Autodesk Inventor part; units mm, degrees
ref_plane "YZ Plane" through (0, 0, 0) normal (1, 0, 0) x (0, 1, 0)
ref_plane "XZ Plane" through (0, 0, 0) normal (0, 1, 0) x (-1, 0, 0)
ref_plane "XY Plane" through (0, 0, 0) normal (0, 0, 1) x (1, 0, 0)
sketch "Sketch1" plane through (0, 0, 0) normal (0, 1, 0) x (-1, 0, 0)
  line L0 (40, 40) -> (-40, 40) construction
  line L1 (-40, 40) -> (-40, -40) construction
  line L2 (-40, -40) -> (40, -40) construction
  line L3 (40, -40) -> (40, 40) construction
  line L4 (-40, 40) -> (40, -40) construction
  line L5 (100, -45) -> (-100, -45)
  line L6 (-100, -45) -> (-100, 100)
  line L7 (-100, 100) -> (100, 100)
  line L8 (100, 100) -> (100, -45)
  circle A0 centre (85, 0) radius 6.5
  circle A1 centre (0, 85) radius 6.5
  circle A2 centre (-85, 0) radius 6.5
  line L9 (0, 40) -> (0, -40) construction
  line L10 (100, 15) -> (20, 100)
  line L11 (-20, 100) -> (-100, 15)
  line L12 (100, -15) -> (71.7647, -45)
  line L13 (-100, -15) -> (-71.7647, -45)
  line L14 (0, 0) -> (-40, 0) construction
  point P0 (0, 0)
  point P1 (0, 0)
  dimension "d2" = 80
  dimension "d3" = 80
  dimension "d17" = 5
  dimension "d18" = 13
  dimension "d19" = 45
  dimension "d20" = 45
  dimension "d21" = 40
  dimension "d22" = 15
  dimension "d23" = 15
  dimension "d24" = 30
extrude "Plate1" add sketch "Sketch1" along normal blind 3 contours L5 L13 L6 L11 L7 L10 L8 L12
fillet "Corner Round2" radius 6 8 edges at (-20, 1.5, 100) (20, 1.5, 100) (100, 1.5, 15) (100, 1.5, -15) (71.7647, 1.5, -45) (-100, 1.5, 15) (-100, 1.5, -15) (-71.7647, 1.5, -45)
equation "\"d20\" = d19"
equation "\"d23\" = d22"
equation "\"BendReliefWidth\" = Thickness"
equation "\"BendReliefDepth\" = 0.5 * Thickness"
equation "\"CornerReliefSize\" = 4 * Thickness"
equation "\"MinimumRemnant\" = 2 * Thickness"
equation "\"TransitionRadius\" = BendRadius"
equation "\"JacobiRadiusSize\" = BendRadius"
equation "\"GapSize\" = Thickness"
properties part number "MSC 907 flange frame heel" material "Stainless Steel"
Input: part model. Units: mm. Frame: model coordinates. Give positions to 0.01 mm unless a question says otherwise; leave off trailing zeros. Order: outer loops, then holes, each group sorted by start corner. A loop starts at its lowest first (then second) coordinate and runs counter-clockwise, first axis right, second up.
Q1. Section B-B on z = 0. Output: boundary loops of the cut face in (x, y), and give its area (3 significant figures).
Checked values:
outline: (-100, 0) - (-91.5, 0) - (-91.5, 3) - (-100, 3) - close; (-78.5, 0) - (78.5, 0) - (78.5, 3) - (-78.5, 3) - close; (91.5, 0) - (100, 0) - (100, 3) - (91.5, 3) - close
area: 522 mm2
Q2. Draft query along Z for faces 1 (the flat face through (-86.129, 1.479, -29.738)), 2 (the flat face through (-60.61, 1.48, 56.85)), 3 (the cylindrical face through (79, 1.5, 2.5)), 4 (the flat face through (1, 3, 12)). Return one class per face: +Z half, -Z half, draft (parallel to the pull), parting line (faces both ways), or undercut.
Checked values:
face 1: -Z half
face 2: +Z half
face 3: undercut
face 4: draft
Q3. Ray query, probe 1 along Z at (x, y) = (0, 2.45); probe 2 along Z at (x, y) = (-85, 0.85); probe 3 along X at (y, z) = (2.25, 88). Return the intervals inside material, ascending.
Checked values:
probe 1: z = -45 to 78.5, 91.5 to 100
probe 2: z = -30.94 to -6.5, 6.5 to 30.94
probe 3: x = -31.29 to -5.77, 5.77 to 31.29
Q4. Section A-A on x = 0. Output: boundary loops of the cut face in (y, z), and give its area (3 significant figures).
Checked values:
outline: (0, -45) - (3, -45) - (3, 78.5) - (0, 78.5) - close; (0, 91.5) - (3, 91.5) - (3, 100) - (0, 100) - close
area: 396 mm2
Q5. Section D-D on z = 32. Output: boundary loops of the cut face in (x, y), and give its area (3 significant figures).
Checked values:
outline: (-84, 0) - (84, 0) - (84, 3) - (-84, 3) - close
area: 504 mm2
Q6. Section C-C on y = 2.5. Output: boundary loops of the cut face in (x, z), and give its area (3 significant figures).
Checked values:
outline: (-100, -12.62) arc R6 ccw to (-98.37, -16.73) - (-73.54, -43.11) arc R6 ccw to (-69.17, -45) - (69.17, -45) arc R6 ccw to (73.54, -43.11) - (98.37, -16.73) arc R6 ccw to (100, -12.62) - (100, 12.62) arc R6 ccw to (98.37, 16.73) - (21.78, 98.11) arc R6 ccw to (17.41, 100) - (-17.41, 100) arc R6 ccw to (-21.78, 98.11) - (-98.37, 16.73) arc R6 ccw to (-100, 12.62) - close; hole circle Ø13 at (-85, 0); hole circle Ø13 at (0, 85); hole circle Ø13 at (85, 0)
area: 20,900 mm2
